Verification items for the finished model (mm, model axes). A direction names the side the tool comes from. Round coordinates to 2 decimals unless told otherwise and drop trailing zeros. Put each result on its own line as item: value.
from build123d import *

# Parameters (mm, degrees)
SKETCH1_R           = 2.1
BOSS_EXTRUDE1_DEPTH = 130


with BuildPart() as part:
    # Sketch1 → Boss-Extrude1 (new body)
    with BuildSketch(Plane.XY):
        with BuildLine():
            Line((-8.5, 10), (-4.862792737, 10))
            ThreePointArc((-4.862792737, 10), (-4.598292737, 9.947387679), (-4.374060464, 9.797560464))
            Line((-4.374060464, 9.797560464), (-3.3865, 8.81))
            Line((-3.3865, 8.81), (-3.3865, 8.2))
            Line((-3.3865, 8.2), (-5.5, 8.2))
            Line((-5.5, 8.2), (-5.5, 6.561))
            Line((-5.5, 6.561), (-2.8395, 3.9005))
            Line((-2.8395, 3.9005), (-0.1, 3.9005))
            Line((-0.1, 3.9005), (0, 3.8005))
            Line((0, 3.8005), (0.1, 3.9005))
            Line((0.1, 3.9005), (2.8395, 3.9005))
            Line((2.8395, 3.9005), (5.5, 6.561))
            Line((5.5, 6.561), (5.5, 8.2))
            Line((5.5, 8.2), (3.3865, 8.2))
            Line((3.3865, 8.2), (3.3865, 8.81))
            Line((3.3865, 8.81), (4.374060464, 9.797560464))
            ThreePointArc((4.374060464, 9.797560464), (4.598292737, 9.947387679), (4.862792737, 10))
            Line((4.862792737, 10), (8.5, 10))
            ThreePointArc((8.5, 10), (9.560660172, 9.560660172), (10, 8.5))
            Line((10, 8.5), (10, 4.862792737))
            ThreePointArc((10, 4.862792737), (9.947387679, 4.598292737), (9.797560464, 4.374060464))
            Line((9.797560464, 4.374060464), (8.81, 3.3865))
            Line((8.81, 3.3865), (8.2, 3.3865))
            Line((8.2, 3.3865), (8.2, 5.5))
            Line((8.2, 5.5), (6.561, 5.5))
            Line((6.561, 5.5), (3.9005, 2.8395))
            Line((3.9005, 2.8395), (3.9005, 0.1))
            Line((3.9005, 0.1), (3.8005, 0))
            Line((3.8005, 0), (3.9005, -0.1))
            Line((3.9005, -0.1), (3.9005, -2.8395))
            Line((3.9005, -2.8395), (6.561, -5.5))
            Line((6.561, -5.5), (8.2, -5.5))
            Line((8.2, -5.5), (8.2, -3.3865))
            Line((8.2, -3.3865), (8.81, -3.3865))
            Line((8.81, -3.3865), (9.797560464, -4.374060464))
            ThreePointArc((9.797560464, -4.374060464), (9.947387679, -4.598292737), (10, -4.862792737))
            Line((10, -4.862792737), (10, -8.5))
            ThreePointArc((10, -8.5), (9.560660172, -9.560660172), (8.5, -10))
            Line((8.5, -10), (4.862792737, -10))
            ThreePointArc((4.862792737, -10), (4.598292737, -9.947387679), (4.374060464, -9.797560464))
            Line((4.374060464, -9.797560464), (3.3865, -8.81))
            Line((3.3865, -8.81), (3.3865, -8.2))
            Line((3.3865, -8.2), (5.5, -8.2))
            Line((5.5, -8.2), (5.5, -6.561))
            Line((5.5, -6.561), (2.8395, -3.9005))
            Line((2.8395, -3.9005), (0.1, -3.9005))
            Line((0.1, -3.9005), (0, -3.8005))
            Line((0, -3.8005), (-0.1, -3.9005))
            Line((-0.1, -3.9005), (-2.8395, -3.9005))
            Line((-2.8395, -3.9005), (-5.5, -6.561))
            Line((-5.5, -6.561), (-5.5, -8.2))
            Line((-5.5, -8.2), (-3.3865, -8.2))
            Line((-3.3865, -8.2), (-3.3865, -8.81))
            Line((-3.3865, -8.81), (-4.374060464, -9.797560464))
            ThreePointArc((-4.374060464, -9.797560464), (-4.598292737, -9.947387679), (-4.862792737, -10))
            Line((-4.862792737, -10), (-8.5, -10))
            ThreePointArc((-8.5, -10), (-9.560660172, -9.560660172), (-10, -8.5))
            Line((-10, -8.5), (-10, -4.862792737))
            ThreePointArc((-10, -4.862792737), (-9.947387679, -4.598292737), (-9.797560464, -4.374060464))
            Line((-9.797560464, -4.374060464), (-8.81, -3.3865))
            Line((-8.81, -3.3865), (-8.2, -3.3865))
            Line((-8.2, -3.3865), (-8.2, -5.5))
            Line((-8.2, -5.5), (-6.561, -5.5))
            Line((-6.561, -5.5), (-3.9005, -2.8395))
            Line((-3.9005, -2.8395), (-3.9005, -0.1))
            Line((-3.9005, -0.1), (-3.8005, 0))
            Line((-3.8005, 0), (-3.9005, 0.1))
            Line((-3.9005, 0.1), (-3.9005, 2.8395))
            Line((-3.9005, 2.8395), (-6.561, 5.5))
            Line((-6.561, 5.5), (-8.2, 5.5))
            Line((-8.2, 5.5), (-8.2, 3.3865))
            Line((-8.2, 3.3865), (-8.81, 3.3865))
            Line((-8.81, 3.3865), (-9.797560464, 4.374060464))
            ThreePointArc((-9.797560464, 4.374060464), (-9.947387679, 4.598292737), (-10, 4.862792737))
            Line((-10, 4.862792737), (-10, 8.5))
            ThreePointArc((-10, 8.5), (-9.560660172, 9.560660172), (-8.5, 10))
        make_face()
        Circle(SKETCH1_R, mode=Mode.SUBTRACT)
    extrude(amount=BOSS_EXTRUDE1_DEPTH)


solid = part.part
Item 1: Material ranges on L1, parallel to Y at x = 0, z = 58; L2, parallel to Y at x = 7.5, z = 61.5, recorded low to high. Write a range as [from, to].
Check sheet entries:
L1: y = [-3.8, -2.1], [2.1, 3.8]
L2: y = [-10, -5.5], [5.5, 10]
Item 2: Release check for a two-part mould opening along Y. For faces 6 (the flat face through (-1, 3.9, 64)), 7 (the flat face through (-7, -10, 64)), 8 (the flat face through (8.2, 4, 64)) record: +Y half, -Y half, draft (parallel to the pull), parting line (faces both ways), or undercut.
Check sheet entries:
face 6: +Y half
face 7: -Y half
face 8: undercut
Item 3: Gauge pin test, flat ends, axial feed: pin 1 Ø4 at (x, z) = (3, 84) entering from -Y; pin 2 Ø1 at (x, z) = (-2, 43) entering from -Y; pin 3 Ø1.4 at (y, z) = (-1.5, 62.5) entering from -X; pin 4 Ø1.5 at (y, z) = (3, 114.5) entering from +X. Record the tip position at first contact, or that the pin passes through.
Check sheet entries:
pin 1: stops at y = -10
pin 2: stops at y = -3.9
pin 3: stops at x = -3.9
pin 4: stops at x = 9.17
Item 4: Tool access check on faces 1 (the flat face through (-8.2, -4, 64)), 2 (the flat face through (1, -3.9, 64)), 3 (the flat face through (3.9, -1, 64)), 4 (the flat face through (7, -10, 64)), 5 (the flat face through (1, 3.9, 64)). Record the directions out of +Z, -Z, +X, -X, +Y, -Y that give a thin tool (end or side, any length) a straight path to the whole face; none if there is none.
Check sheet entries:
face 1: +Z, -Z
face 2: +Z, -Z, -Y
face 3: +Z, -Z, +X
face 4: +Z, -Z, +X, -X, -Y
face 5: +Z, -Z, +Y
